from build123d import *

# Parameters (mm, degrees)
SKETCH1_R           = 101.859163579
SKETCH1_R_2         = 2
SKETCH1_R_3         = 10
BOSS_EXTRUDE1_DEPTH = 3


with BuildPart() as part:
    # Sketch1 → Boss-Extrude1 (new body)
    with BuildSketch(Plane.XY):
        Circle(SKETCH1_R)
        with Locations((0, 30)):
            Circle(SKETCH1_R_2, mode=Mode.SUBTRACT)
        with Locations((-10, 50)):
            Circle(SKETCH1_R_2, mode=Mode.SUBTRACT)
        with Locations((0, 40)):
            Circle(SKETCH1_R_2, mode=Mode.SUBTRACT)
        with Locations((10, 50)):
            Circle(SKETCH1_R_2, mode=Mode.SUBTRACT)
        with Locations((-10, 60)):
            Circle(SKETCH1_R_2, mode=Mode.SUBTRACT)
        with Locations((-10, 40)):
            Circle(SKETCH1_R_2, mode=Mode.SUBTRACT)
        with Locations((10, 40)):
            Circle(SKETCH1_R_2, mode=Mode.SUBTRACT)
        with Locations((0, 50)):
            Circle(SKETCH1_R_2, mode=Mode.SUBTRACT)
        with Locations((10, 60)):
            Circle(SKETCH1_R_2, mode=Mode.SUBTRACT)
        with Locations((-10, 70)):
            Circle(SKETCH1_R_2, mode=Mode.SUBTRACT)
        with Locations((0, 60)):
            Circle(SKETCH1_R_2, mode=Mode.SUBTRACT)
        with Locations((10, 70)):
            Circle(SKETCH1_R_2, mode=Mode.SUBTRACT)
        with Locations((-10, 80)):
            Circle(SKETCH1_R_2, mode=Mode.SUBTRACT)
        with Locations((0, 70)):
            Circle(SKETCH1_R_2, mode=Mode.SUBTRACT)
        with Locations((10, 80)):
            Circle(SKETCH1_R_2, mode=Mode.SUBTRACT)
        with Locations((25.980762114, -15)):
            Circle(SKETCH1_R_2, mode=Mode.SUBTRACT)
        with Locations((48.301270189, -16.339745962)):
            Circle(SKETCH1_R_2, mode=Mode.SUBTRACT)
        with Locations((34.641016151, -20)):
            Circle(SKETCH1_R_2, mode=Mode.SUBTRACT)
        with Locations((38.301270189, -33.660254038)):
            Circle(SKETCH1_R_2, mode=Mode.SUBTRACT)
        with Locations((56.961524227, -21.339745962)):
            Circle(SKETCH1_R_2, mode=Mode.SUBTRACT)
        with Locations((39.641016151, -11.339745962)):
            Circle(SKETCH1_R_2, mode=Mode.SUBTRACT)
        with Locations((29.641016151, -28.660254038)):
            Circle(SKETCH1_R_2, mode=Mode.SUBTRACT)
        with Locations((43.301270189, -25)):
            Circle(SKETCH1_R_2, mode=Mode.SUBTRACT)
        with Locations((46.961524227, -38.660254038)):
            Circle(SKETCH1_R_2, mode=Mode.SUBTRACT)
        with Locations((65.621778265, -26.339745962)):
            Circle(SKETCH1_R_2, mode=Mode.SUBTRACT)
        with Locations((51.961524227, -30)):
            Circle(SKETCH1_R_2, mode=Mode.SUBTRACT)
        with Locations((55.621778265, -43.660254038)):
            Circle(SKETCH1_R_2, mode=Mode.SUBTRACT)
        with Locations((74.282032303, -31.339745962)):
            Circle(SKETCH1_R_2, mode=Mode.SUBTRACT)
        with Locations((60.621778265, -35)):
            Circle(SKETCH1_R_2, mode=Mode.SUBTRACT)
        with Locations((64.282032303, -48.660254038)):
            Circle(SKETCH1_R_2, mode=Mode.SUBTRACT)
        with Locations((-25.980762114, -15)):
            Circle(SKETCH1_R_2, mode=Mode.SUBTRACT)
        with Locations((-38.301270189, -33.660254038)):
            Circle(SKETCH1_R_2, mode=Mode.SUBTRACT)
        with Locations((-34.641016151, -20)):
            Circle(SKETCH1_R_2, mode=Mode.SUBTRACT)
        with Locations((-48.301270189, -16.339745962)):
            Circle(SKETCH1_R_2, mode=Mode.SUBTRACT)
        with Locations((-46.961524227, -38.660254038)):
            Circle(SKETCH1_R_2, mode=Mode.SUBTRACT)
        with Locations((-29.641016151, -28.660254038)):
            Circle(SKETCH1_R_2, mode=Mode.SUBTRACT)
        with Locations((-39.641016151, -11.339745962)):
            Circle(SKETCH1_R_2, mode=Mode.SUBTRACT)
        with Locations((-43.301270189, -25)):
            Circle(SKETCH1_R_2, mode=Mode.SUBTRACT)
        with Locations((-56.961524227, -21.339745962)):
            Circle(SKETCH1_R_2, mode=Mode.SUBTRACT)
        with Locations((-55.621778265, -43.660254038)):
            Circle(SKETCH1_R_2, mode=Mode.SUBTRACT)
        with Locations((-51.961524227, -30)):
            Circle(SKETCH1_R_2, mode=Mode.SUBTRACT)
        with Locations((-65.621778265, -26.339745962)):
            Circle(SKETCH1_R_2, mode=Mode.SUBTRACT)
        with Locations((-64.282032303, -48.660254038)):
            Circle(SKETCH1_R_2, mode=Mode.SUBTRACT)
        with Locations((-60.621778265, -35)):
            Circle(SKETCH1_R_2, mode=Mode.SUBTRACT)
        with Locations((-74.282032303, -31.339745962)):
            Circle(SKETCH1_R_2, mode=Mode.SUBTRACT)
        with Locations((77.942286341, 45)):
            Circle(SKETCH1_R_2, mode=Mode.SUBTRACT)
        with Locations((77.942286341, -45)):
            Circle(SKETCH1_R_2, mode=Mode.SUBTRACT)
        with Locations((0, -90)):
            Circle(SKETCH1_R_2, mode=Mode.SUBTRACT)
        with Locations((-77.942286341, -45)):
            Circle(SKETCH1_R_2, mode=Mode.SUBTRACT)
        with Locations((-77.942286341, 45)):
            Circle(SKETCH1_R_2, mode=Mode.SUBTRACT)
        with Locations((0, 90)):
            Circle(SKETCH1_R_2, mode=Mode.SUBTRACT)
        Circle(SKETCH1_R_3, mode=Mode.SUBTRACT)
        with Locations((25.980762114, 15)):
            Circle(SKETCH1_R_2, mode=Mode.SUBTRACT)
        with Locations((0, -30)):
            Circle(SKETCH1_R_2, mode=Mode.SUBTRACT)
        with Locations((-25.980762114, 15)):
            Circle(SKETCH1_R_2, mode=Mode.SUBTRACT)
    extrude(amount=BOSS_EXTRUDE1_DEPTH)


solid = part.part
Here's how the part is built. I have some questions about the finished solid (model axes, mm). Round coordinates to 2 decimals unless told otherwise and drop trailing zeros. Order: outer loops, then holes, each group sorted by start corner. A loop starts at its lowest first (then second) coordinate and runs counter-clockwise, first axis right, second up. Notation, with made-up numbers: M -11,-19.5 L 37,-19.5 A11 cw 37,-0.5 Z; hole C -4.75,21.5 d8. An arc over 180 degrees is marked long. Return JSON: item names as keys, results as strings. Group by question number.
1. If we mould it in two halves opening along X, with no side actions, what happens to faces 1 (the face through (-2.17, -9.76, 1.48)), 2 (the face through (21, 1, 0)), 3 (the face through (-13.26, 100.992, 1.479))? For each: pulls with the +X half, pulls with the -X half, needs draft (parallel to the pull), parting line crosses it, or undercut.
2. If we section it at B-B on z = 2.45: State how many separate pieces and enclosed holes the cut face has, then the cut area to 3 significant figures.
3. If we section it at A-A on x = 5: List the corners of the cut face in (y, z) for me.
4. Please list where these lines run through material, in increasing order: probe 1 along Y at (x, z) = (40, 0.45); probe 2 along Y at (x, z) = (-38, 0.4); probe 3 along X at (y, z) = (-21.5, 0.6).
5. I'm going to push flat-ended pins straight in: pin 1 Ø3 at (x, y) = (-46.96, -38.66) entering from -Z; pin 2 Ø1 at (y, z) = (47.5, 0.5) entering from -X. Where does each tip first touch, or does it pass through?
Reply:
{
 "1": {"face 1": "undercut", "face 2": "needs draft", "face 3": "parting line crosses it"},
 "2": {"separate pieces": "1", "enclosed holes": "55", "area": "31,600 mm^2"},
 "3": {"outline": "M -101.74,0 L -8.66,0 L -8.66,3 L -101.74,3 Z; M 8.66,0 L 101.74,0 L 101.74,3 L 8.66,3 Z"},
 "4": {"probe 1": "-93.68 to -34.72, -32.6 to -13.31, -9.37 to 93.68", "probe 2": "-94.51 to -35.64, -31.68 to -12.48, -10.2 to 94.51", "probe 3": "-99.56 to -58.96, -54.97 to -35.96, -33.32 to 33.32, 35.96 to 54.97, 58.96 to 99.56"},
 "5": {"pin 1": "through", "pin 2": "x = -90.37"}
}
